Geometry check sheet. Reference: the model listing, model coordinates, mm. Round coordinates to 2 decimals unless told otherwise and drop trailing zeros. Loops run counter-clockwise (first coordinate to the right, second up) from the corner with the lowest first, then second, coordinate; pieces in that order, holes last. Notation, with made-up numbers: M 81.25,47 L 126.25,47 A8 ccw 126.25,62 Z; hole C 18,30.5 d11. An arc over 180 degrees is marked long. Answer in a Markdown table with one row per item. Add a question column.
Autodesk Inventor part; units mm, degrees
ref_plane "YZ Plane" through (0, 0, 0) normal (1, 0, 0) x (0, 1, 0)
ref_plane "XZ Plane" through (0, 0, 0) normal (0, 1, 0) x (-1, 0, 0)
ref_plane "XY Plane" through (0, 0, 0) normal (0, 0, 1) x (1, 0, 0)
sketch "Sketch1" plane through (0, 0, 0) normal (0, 0, 1) x (1, 0, 0)
  line L0 (-12.7, 12.7) -> (12.7, 12.7)
  line L1 (12.7, 12.7) -> (12.7, -12.7)
  line L2 (12.7, -12.7) -> (-12.7, -12.7)
  line L3 (-12.7, -12.7) -> (-12.7, 12.7)
  line L4 (-12.7, 12.7) -> (12.7, -12.7) construction
  line L5 (12.7, 12.7) -> (-12.7, -12.7) construction
  point P0 (0, 0)
  dimension "d0" = 25.4
  dimension "d1" = 25.4
extrude "Extrusion1" add sketch "Sketch1" along normal blind 88.9
shell "Shell1" thickness 1.9844 removed faces 2 at (4.2333, -4.2333, 0) at (4.2333, -4.2333, 88.9)
sketch "Sketch2" plane through (-12.7, -12.7, 0) normal (-1, 0, 0) x (0, 0, 1)
  circle A0 centre (19.0501, 12.7399) radius 3.175
  circle A1 centre (31.7501, 12.7399) radius 3.175
  line L0 (0, 12.7) -> (88.9, 12.7) construction
  circle A2 centre (44.45, 12.7) radius 3.175
  circle A3 centre (57.15, 12.7) radius 3.175
  circle A4 centre (69.85, 12.7) radius 3.175
  circle A5 centre (82.55, 12.7) radius 3.175
  line L1 (0, 25.4) -> (88.9, 25.4) construction
  line L2 (44.45, 25.4) -> (44.45, 0) construction
  circle A6 centre (6.3501, 12.7) radius 3.175
  dimension "d5" = 6.35
  dimension "d6" = 6.35
  dimension "d7" = 6.35
  dimension "d8" = 6.35
  dimension "d9" = 6.35
  dimension "d10" = 6.35
  dimension "d11" = 12.7
  dimension "d12" = 12.7
  dimension "d13" = 12.7
  dimension "d14" = 12.7
  dimension "d15" = 12.7
  dimension "d16" = 6.35
  dimension "d17" = 12.7
extrude "Extrusion2" cut sketch "Sketch2" against normal blind 88.9
sketch "Sketch3" plane through (-12.7, 12.7, 0) normal (0, 1, 0) x (1, 0, 0)
  line L0 (23.4156, -47.625) -> (25.4, -47.625) construction
  circle A0 centre (12.7, -44.45) radius 3.175
  circle A1 centre (12.7, -31.75) radius 3.175
  circle A2 centre (12.7, -19.05) radius 3.175
  circle A3 centre (12.7, -6.35) radius 3.175
  line L1 (12.7, 0) -> (12.7, -88.9) construction
  line L2 (0, -88.9) -> (25.4, -88.9) construction
  line L3 (25.4, -44.45) -> (0, -44.45) construction
  line L4 (0, -47.625) -> (0, -41.275) construction
  circle A4 centre (12.7, -57.15) radius 3.175
  circle A5 centre (12.7, -69.85) radius 3.175
  circle A6 centre (12.7, -82.55) radius 3.175
  line L5 (12.7, -88.9) -> (12.7, 0) construction
  dimension "d20" = 6.35
  dimension "d21" = 6.35
  dimension "d22" = 6.35
  dimension "d23" = 6.35
  dimension "d25" = 12.7
  dimension "d26" = 12.7
  dimension "d27" = 12.7
extrude "Extrusion3" cut sketch "Sketch3" against normal blind 88.9
equation "\"d6\" = d5"
equation "\"d7\" = d5"
equation "\"d8\" = d5"
equation "\"d9\" = d5"
equation "\"d10\" = d5"
equation "\"d12\" = d11"
equation "\"d13\" = d11"
equation "\"d14\" = d11"
equation "\"d15\" = d11"
equation "\"d16\" = d5"
equation "\"d17\" = d11"
equation "\"d21\" = d20"
equation "\"d22\" = d20"
equation "\"d23\" = d20"
equation "\"d26\" = d25"
equation "\"d27\" = d25"
properties part number "SquareTube"
1) Cross-section at A-A, the plane y = -7. Record the boundary of the cut face in (x, z).
2) Thickness scan on L1, parallel to Y at x = 4.25, z = 71; L2, parallel to X at y = -11.15, z = 69.85 (3 decimals). Record the ranges inside material, lowest first. Write a range as [from, to].
3) Go/stop test with flat-tipped pins: pin 1 (8.5 mm diameter, centred on x = 0, z = 19.05, fed in from +Y); pin 2 (4 mm diameter, centred on y = 0, z = 69.85, fed in from -X). Record where each tip stops, or that it passes through.
4) Cross-section at D-D, the plane x = 0. Count the separate pieces of the cut face and the enclosed holes in it, plus the area to 3 significant figures.
5) Draft check along X on faces 1 (the flat face through (11, 0, 88.9)), 2 (the flat face through (-10.716, -5, 44)), 3 (the flat face through (-12.7, 5, 44)). Enter one of: +X half, -X half, draft (parallel to the pull), parting line (faces both ways), or undercut.
6) Cross-section at C-C, the plane z = 63.5. Record the boundary of the cut face in (x, y).
Worked answers:
| question | item | result |
|---|---|---|
| 1 | outline | M -12.7,0 L -10.72,0 L -10.72,88.9 L -12.7,88.9 Z; M 10.72,0 L 12.7,0 L 12.7,88.9 L 10.72,88.9 Z |
| 2 | L1 | y = [-12.7, -10.72], [10.72, 12.7] |
| 2 | L2 | x = [-12.7, -3.175], [3.175, 12.7] |
| 3 | pin 1 | stops at y = 12.7 |
| 3 | pin 2 | passes through |
| 4 | separate pieces | 16 |
| 4 | enclosed holes | 0 |
| 4 | area | 176 mm2 |
| 5 | face 1 | draft |
| 5 | face 2 | undercut |
| 5 | face 3 | -X half |
| 6 | outline | M -12.7,-12.7 L 12.7,-12.7 L 12.7,12.7 L -12.7,12.7 Z; hole M -10.72,-10.72 L 10.72,-10.72 L 10.72,10.72 L -10.72,10.72 Z |
